```python
from build123d import *

# Parameters (mm, degrees)
CROQUIS1_W              = 235
CROQUIS1_H              = 70
SALIENTE_EXTRUIR1_DEPTH = 8
CROQUIS2_W              = 235
CROQUIS2_H              = 49.698460378
SALIENTE_EXTRUIR2_DEPTH = 8
SALIENTE_EXTRUIR3_DEPTH = 300
CROQUIS4_W              = 235
CROQUIS4_H              = 9.525
SALIENTE_EXTRUIR4_DEPTH = 40


with BuildPart() as part:
    # Croquis1 → Saliente-Extruir1 (new body)
    with BuildSketch(Plane.XY):
        Rectangle(CROQUIS1_W, CROQUIS1_H)
    extrude(amount=SALIENTE_EXTRUIR1_DEPTH)

    # Croquis2 → Saliente-Extruir2 (add)
    with BuildSketch(Plane(origin=(0, 35, 0), x_dir=(1, 0, 0), z_dir=(0, 1, 0))):
        with Locations((0, -24.849230189)):
            Rectangle(CROQUIS2_W, CROQUIS2_H)
    extrude(amount=-SALIENTE_EXTRUIR2_DEPTH)

    # Croquis3 → Saliente-Extruir3 (add)
    with BuildSketch(Plane(origin=(0, 0, 0), x_dir=(-1, 0, 0), z_dir=(0, 0, -1))):
        Polygon((-117.5, 35), (-117.5, 60.4), (-111.15, 60.4), (-111.15, 41.35), (-92.1, 41.35), (-92.1, 35), align=None)
        Polygon((57.1, 35), (82.5, 35), (82.5, 60.4), (76.15, 60.4), (76.15, 41.35), (57.1, 41.35), align=None)
    extrude(amount=-SALIENTE_EXTRUIR3_DEPTH)

    # Croquis4 → Saliente-Extruir4 (add)
    with BuildSketch(Plane.XY.offset(8)):
        with Locations((0, -30.2375)):
            Rectangle(CROQUIS4_W, CROQUIS4_H)
    extrude(amount=SALIENTE_EXTRUIR4_DEPTH)


solid = part.part
```
Build history of the part. All positions in model axes, mm. A direction names the side the tool comes from. Round coordinates to 2 decimals unless told otherwise and drop trailing zeros. Write each loop counter-clockwise with the first axis right and the second up, starting at its lowest first coordinate (ties: lowest second). Pieces come first, ordered by that corner, then holes.
1) Band-saw the part on C-C, the plane z = 218.5. List the corners of the cut face in (x, y).
2) 3-axis set-ups, long thin cutter, end or side, ignore diameter. For faces 1 (the flat face through (-2, 27, 29)), 2 (the flat face through (102, 41.35, 148)), 3 (the flat face through (105, 35, 173)): which of +Z, -Z, +X, -X, +Y, -Y reach the whole face in a straight line?
3) Band-saw the part on D-D, the plane y = 19.5. List the corners of the cut face in (x, z), and give its area (3 significant figures).
4) Drill centre lines: probe 1 along X at (y, z) = (56.5, 131); probe 2 along Y at (x, z) = (63, 23.5) (3 decimals); probe 3 along X at (y, z) = (37, 233). Where is each one in solid material? Low to high.
5) Band-saw the part on A-A, the plane z = 28. List the corners of the cut face in (x, y) (3 decimals).
6) Pin check, flat tips, straight feed: pin 1 (10.5 mm diameter, centred on x = 16.5, y = -28.5, fed in from +Z); pin 2 (6.5 mm diameter, centred on x = -42.5, y = 30, fed in from +Z); pin 3 (20.5 mm diameter, centred on x = 111, z = 233, fed in from -Y). Stop position of each tip, or through.
7) Band-saw the part on B-B, the plane x = -63. List the corners of the cut face in (y, z) (3 decimals), and give its area (3 significant figures).
Ans:
1. outline: (-82.5, 35) - (-57.1, 35) - (-57.1, 41.35) - (-76.15, 41.35) - (-76.15, 60.4) - (-82.5, 60.4) - close; (92.1, 35) - (117.5, 35) - (117.5, 60.4) - (111.15, 60.4) - (111.15, 41.35) - (92.1, 41.35) - close
2. face 1: +Z, +X, -X
2. face 2: +Z, -Z, +Y
2. face 3: +Z, +X, -X, -Y
3. outline: (-117.5, 0) - (117.5, 0) - (117.5, 8) - (-117.5, 8) - close
3. area: 1,880 mm2
4. probe 1: x = -82.5 to -76.15, 111.15 to 117.5
4. probe 2: y = -35 to -25.475, 27 to 35
4. probe 3: x = -82.5 to -57.1, 92.1 to 117.5
5. outline: (-117.5, -35) - (117.5, -35) - (117.5, -25.475) - (-117.5, -25.475) - close; (-117.5, 27) - (117.5, 27) - (117.5, 60.4) - (111.15, 60.4) - (111.15, 41.35) - (92.1, 41.35) - (92.1, 35) - (-57.1, 35) - (-57.1, 41.35) - (-76.15, 41.35) - (-76.15, 60.4) - (-82.5, 60.4) - (-82.5, 35) - (-117.5, 35) - close
6. pin 1: stops at z = 48
6. pin 2: stops at z = 49.7
6. pin 3: stops at y = 35
7. outline: (-35, 0) - (41.35, 0) - (41.35, 300) - (35, 300) - (35, 49.698) - (27, 49.698) - (27, 8) - (-25.475, 8) - (-25.475, 48) - (-35, 48) - close
7. area: 3,180 mm2
